Read the model definition and answer for the solid it produces. Units are mm, in the model's axes. A direction names the side the tool comes from. Coordinates: 2 decimals unless noted, no trailing zeros. Write each loop counter-clockwise with the first axis right and the second up, starting at its lowest first coordinate (ties: lowest second). Pieces come first, ordered by that corner, then holes.
(1) Straight lines are drawn through the part: line 1 along Z through (x, y) = (5.5, -1); line 2 along Y through (x, z) = (-0.5, 180.5); line 3 along Z through (x, y) = (-5, 30.5). For each, find the intervals that lie inside material, in ascending order.
(2) The part is cut by section D-D, the plane x = -8.5. Determine the outline of the cut face in (y, z).
(3) The part is cut by section C-C, the plane z = 71.5. Determine the outline of the cut face in (x, y), and give its area (3 significant figures).
(4) Given pin 1 (12 mm diameter, centred on y = -24, z = 74, fed in from -X); pin 2 (12 mm diameter, centred on y = -8, z = 130, fed in from -X); pin 3 (2 mm diameter, centred on x = 16.5, z = 92.5, fed in from -Y), each flat-ended and moving along its own axis, determine where each tip first touches the part or whether it passes through.
(5) The part is cut by section A-A, the plane y = 0. Determine the outline of the cut face in (x, z).
(6) Which of the six approach directions +Z, -Z, +X, -X, +Y, -Y give full straight-line access (tool end or side, diameter ignored) to faces 1 (the cylindrical face through (-12.69, 24.397, 115.978)), 2 (the cylindrical face through (28, -21, 34)), 3 (the cylindrical face through (-12.69, 24.397, 16.902))?
```python
from build123d import *

# Parameters (mm, degrees)
SKETCH1_R                = 5
BOSS_EXTRUDE1_DEPTH      = 10
SKETCH2_R                = 27.5
BOSS_EXTRUDE2_DEPTH      = 180
BOSS_EXTRUDE3_DEPTH      = 10
BOSS_EXTRUDE3_DEPTH_BACK = 10
SKETCH3_R                = 35
SKETCH5_R                = 5
BOSS_EXTRUDE4_DEPTH      = 20


with BuildPart() as part:
    # Sketch1 → Boss-Extrude1 (new body)
    with BuildSketch(Plane.XY):
        Circle(SKETCH1_R)
    extrude(amount=BOSS_EXTRUDE1_DEPTH)

    # Sketch2 → Boss-Extrude2 (add)
    with BuildSketch(Plane.XY.offset(10)):
        with Locations(Location((0, 0, 0), (0, 0, 180))):
            Circle(SKETCH2_R)
    extrude(amount=BOSS_EXTRUDE2_DEPTH)

    # Sketch3 → Boss-Extrude3 (add, two sides: drawn at the far end of the back side and taken through both)
    with BuildSketch(Plane(origin=(0, 0, 34), x_dir=(-1, 0, 0), z_dir=(0, 0, -1)).offset(-BOSS_EXTRUDE3_DEPTH_BACK)):
        Circle(SKETCH3_R)
    extrude(amount=BOSS_EXTRUDE3_DEPTH + BOSS_EXTRUDE3_DEPTH_BACK)

    # Sketch5 → Boss-Extrude4 (add)
    with BuildSketch(Plane.XY.offset(190)):
        Circle(SKETCH5_R)
    extrude(amount=BOSS_EXTRUDE4_DEPTH)


solid = part.part
```
Computed:
1. line 1: z = 10 to 190
1. line 2: y = -27.5 to 27.5
1. line 3: z = 24 to 44
2. outline: (-33.95, 24) - (-26.15, 24) - (-26.15, 10) - (26.15, 10) - (26.15, 24) - (33.95, 24) - (33.95, 44) - (26.15, 44) - (26.15, 190) - (-26.15, 190) - (-26.15, 44) - (-33.95, 44) - close
3. outline: circle Ø55 at (0, 0)
3. area: 2,380 mm2
4. pin 1: stops at x = -20.79
4. pin 2: stops at x = -27.43
4. pin 3: stops at y = -22.72
5. outline: (-35, 24) - (-27.5, 24) - (-27.5, 10) - (-5, 10) - (-5, 0) - (5, 0) - (5, 10) - (27.5, 10) - (27.5, 24) - (35, 24) - (35, 44) - (27.5, 44) - (27.5, 190) - (5, 190) - (5, 210) - (-5, 210) - (-5, 190) - (-27.5, 190) - (-27.5, 44) - (-35, 44) - close
6. face 1: +Z
6. face 2: +Z, -Z
6. face 3: -Z
